Here's how the part is built. I have some questions about the finished solid (model axes, mm). A direction names the side the tool comes from. Round coordinates to 2 decimals unless told otherwise and drop trailing zeros. Order: outer loops, then holes, each group sorted by start corner. A loop starts at its lowest first (then second) coordinate and runs counter-clockwise, first axis right, second up. Notation, with made-up numbers: (85.5, -31) -> (138.5, -31) arc R23 cw to (138.5, -6) -> close; hole circle Ø8 at (58.25, -32). An arc over 180 degrees is marked (long way). Use a Markdown table: item, result. Add a question column.
Autodesk Inventor part; units mm, degrees
ref_plane "YZ Plane" through (0, 0, 0) normal (1, 0, 0) x (0, 1, 0)
ref_plane "XZ Plane" through (0, 0, 0) normal (0, 1, 0) x (-1, 0, 0)
ref_plane "XY Plane" through (0, 0, 0) normal (0, 0, 1) x (1, 0, 0)
sketch "Sketch1" plane through (0, 0, 0) normal (0, 0, 1) x (1, 0, 0)
  circle A0 centre (0, 0) radius 3.75
  line L0 (1.25, -6.25) -> (-1.25, -6.25)
  line L1 (-1.25, -6.25) -> (-1.25, 6.25) construction
  line L2 (-1.25, 6.25) -> (1.25, 6.25)
  line L3 (1.25, 6.25) -> (1.25, -6.25) construction
  circle A1 centre (0, 0) radius 5.25
  line L4 (1.25, -5.099) -> (1.25, -6.25)
  line L5 (-1.25, -6.25) -> (-1.25, -5.099)
  line L6 (-1.25, 6.25) -> (-1.25, 5.099)
  line L7 (1.25, 6.25) -> (1.25, 5.099)
  arc A2 (-1.25, -5.099) -> (1.25, -5.099) centre (0, 0) ccw
  arc A3 (1.25, 5.099) -> (-1.25, 5.099) centre (0, 0) ccw
  point P0 (0, 6.25)
  point P1 (1.25, 0)
  dimension "d1" = 7.5
  dimension "d10" = 2.5
  dimension "d11" = 12.5
  dimension "d12" = 10.5
extrude "Extrusion1" add sketch "Sketch1" along normal blind 12
sketch "Sketch5" plane through (0, 0, 0) normal (0, 0, -1) x (-1, 0, 0)
  circle A0 centre (0, 0) radius 3.75
  circle A1 centre (0, 0) radius 3.75
  line L0 (-1.25, -6.25) -> (-1.25, -5.099)
  line L1 (1.25, -6.25) -> (-1.25, -6.25)
  line L2 (1.25, -5.099) -> (1.25, -6.25)
  arc A2 (1.25, -5.099) -> (1.25, 5.099) centre (0, 0) ccw
  line L3 (1.25, 6.25) -> (1.25, 5.099)
  line L4 (-1.25, 6.25) -> (1.25, 6.25)
  line L5 (-1.25, 5.099) -> (-1.25, 6.25)
  arc A3 (-1.25, 5.099) -> (-1.25, -5.099) centre (0, 0) ccw
  circle A4 centre (0, 0) radius 1.5
  dimension "d13" = 3
extrude "Extrusion4" add sketch "Sketch5" along normal blind 2 contours A0 | L0 A3 L5 L4 L3 A2 L2 L1
sketch "Sketch6" plane through (0, 0, 0) normal (0, 0, 1) x (1, 0, 0)
  line L0 (0.625, 6.25) -> (-0.625, 6.25)
  line L1 (-0.625, 6.25) -> (-0.625, -6.25) construction
  line L2 (-0.625, -6.25) -> (0.625, -6.25)
  line L3 (0.625, -6.25) -> (0.625, 6.25) construction
  line L4 (-1.25, 6.25) -> (1.25, 6.25)
  circle A0 centre (0, 0) radius 1.5 construction
  arc A1 (0.625, 1.3636) -> (-0.625, 1.3636) centre (0, 0) ccw
  arc A2 (-0.625, -1.3636) -> (0.625, -1.3636) centre (0, 0) ccw
  line L5 (0.625, 6.25) -> (0.625, 1.3636)
  line L6 (-0.625, 6.25) -> (-0.625, 1.3636)
  line L7 (0.625, -1.3636) -> (0.625, -6.25)
  line L8 (-0.625, -1.3636) -> (-0.625, -6.25)
  point P0 (0, 0)
  point P1 (0, 6.25)
  point P2 (0.625, 0)
  dimension "d16" = 1.25
extrude "Extrusion5" add sketch "Sketch6" along normal blind 2
properties part number "AA042" material "ABS Plastic"
(1) I'm going to push flat-ended pins straight in: P1, Ø1.6, axis at y = 3, z = 0.5, coming from the -X side; P2, Ø1, axis at x = 0, y = -3, coming from the +Z side; P3, Ø5, axis at y = -4.5, z = 0.5, coming from the -X side. Where does each tip first touch, or does it pass through?
(2) On a 3-axis mill with a long thin cutter (end or side, diameter ignored), from which of +Z, -Z, +X, -X, +Y, -Y can I reach the whole of each face in a straight line? I mean faces 4 (the cylindrical face through (0, -1.5, 1)), 5 (the flat face through (-0.625, 3, 1)), 6 (the flat face through (-1.25, -6, 5)), 7 (the flat face through (-1.25, 6, 5)). Say none if no direction works.
(3) I want a section at A-A on y = 0. List the corners of the cut face in (x, z) for me.
(4) If we mould it in two halves opening along X, with no side actions, what happens to faces 1 (the cylindrical face through (-5.25, -0.1, 5.92)), 2 (the flat face through (-0.625, -3, 1)), 3 (the flat face through (1.25, 6, 5))? For each: pulls with the +X half, pulls with the -X half, needs draft (parallel to the pull), parting line crosses it, or undercut.
(5) Please list where these lines run through material, in increasing order: probe 1 along Y at (x, z) = (0, -1.1); probe 2 along X at (y, z) = (0, 5.5); probe 3 along Y at (x, z) = (0, 9). Write a range as from..to.
(6) I want a section at B-B on z = 9.75. List the corners of the cut face in (x, y) for me.
(7) I want a section at D-D on z = 1.25. List the corners of the cut face in (x, y) for me (3 decimals), and give its area (3 significant figures).
(8) I want a section at C-C on x = 0. List the corners of the cut face in (y, z) for me, and give its area (3 significant figures).
Output:
| question | item | result |
|---|---|---|
| 1 | P1 | x = -4.77 |
| 1 | P2 | z = 2 |
| 1 | P3 | x = -4.85 |
| 2 | face 4 | +Z, -Z |
| 2 | face 5 | +Z |
| 2 | face 6 | +Z, -Z, -X, -Y |
| 2 | face 7 | +Z, -Z, -X, +Y |
| 3 | outline | (-5.25, -2) -> (-1.5, -2) -> (-1.5, 0) -> (-3.75, 0) -> (-3.75, 12) -> (-5.25, 12) -> close; (1.5, -2) -> (5.25, -2) -> (5.25, 12) -> (3.75, 12) -> (3.75, 0) -> (1.5, 0) -> close |
| 4 | face 1 | pulls with the -X half |
| 4 | face 2 | undercut |
| 4 | face 3 | pulls with the +X half |
| 5 | probe 1 | -6.25..-1.5, 1.5..6.25 |
| 5 | probe 2 | -5.25..-3.75, 3.75..5.25 |
| 5 | probe 3 | -6.25..-3.75, 3.75..6.25 |
| 6 | outline | (-1.25, -6.25) -> (1.25, -6.25) -> (1.25, -5.1) arc R5.25 ccw to (1.25, 5.1) -> (1.25, 6.25) -> (-1.25, 6.25) -> (-1.25, 5.1) arc R5.25 ccw to (-1.25, -5.1) -> close; hole circle Ø7.5 at (0, 0) |
| 7 | outline | (-1.25, -6.25) -> (1.25, -6.25) -> (1.25, -5.099) arc R5.25 ccw to (1.25, 5.099) -> (1.25, 6.25) -> (-1.25, 6.25) -> (-1.25, 5.099) arc R5.25 ccw to (-1.25, -5.099) -> close; hole (-0.625, -3.698) -> (-0.625, -1.364) arc R1.5 ccw to (0.625, -1.364) -> (0.625, -3.698) arc R3.75 ccw to (0.625, 3.698) -> (0.625, 1.364) arc R1.5 ccw to (-0.625, 1.364) -> (-0.625, 3.698) arc R3.75 ccw to start |
| 7 | area | 53.4 mm² |
| 8 | outline | (-6.25, -2) -> (-1.5, -2) -> (-1.5, 2) -> (-3.75, 2) -> (-3.75, 12) -> (-6.25, 12) -> close; (1.5, -2) -> (6.25, -2) -> (6.25, 12) -> (3.75, 12) -> (3.75, 2) -> (1.5, 2) -> close |
| 8 | area | 88.0 mm² |
